Here's how the part is built. I have some questions about the finished solid (model axes, mm). A direction names the side the tool comes from. Give positions to 0.01 mm unless a question says otherwise; leave off trailing zeros. Loops run counter-clockwise (first coordinate to the right, second up) from the corner with the lowest first, then second, coordinate; pieces in that order, holes last. Notation, with made-up numbers: (5, -14) - (47, -14) arc R24 ccw to (47, -3) - close; hole circle Ø3 at (9.5, -26). An arc over 180 degrees is marked (long way). Use a Markdown table: item, result.
Autodesk Inventor part; units mm, degrees
ref_plane "YZ Plane" through (0, 0, 0) normal (1, 0, 0) x (0, 1, 0)
ref_plane "XZ Plane" through (0, 0, 0) normal (0, 1, 0) x (-1, 0, 0)
ref_plane "XY Plane" through (0, 0, 0) normal (0, 0, 1) x (1, 0, 0)
sketch "Sketch1" plane through (0, 0, 0) normal (0, 1, 0) x (-1, 0, 0)
  line L0 (0, 0) -> (11.684, 0)
  line L1 (11.684, 0) -> (11.684, -6.096)
  line L2 (11.684, -6.096) -> (0, -6.096)
  line L3 (0, -6.096) -> (0, -17.78)
  line L4 (0, -17.78) -> (-6.096, -17.78)
  line L5 (-6.096, -17.78) -> (-6.096, -6.096)
  line L6 (-6.096, -6.096) -> (-17.78, -6.096)
  line L7 (-17.78, -6.096) -> (-17.78, 0)
  line L8 (-17.78, 0) -> (-6.096, 0)
  line L9 (-6.096, 0) -> (-6.096, 11.684)
  line L10 (-6.096, 11.684) -> (0, 11.684)
  line L11 (0, 11.684) -> (0, 0)
  arc A0 (11.684, -6.096) -> (11.684, 0) centre (11.684, -3.048) ccw
  arc A1 (-6.096, -17.78) -> (0, -17.78) centre (-3.048, -17.78) ccw
  arc A2 (-17.78, 0) -> (-17.78, -6.096) centre (-17.78, -3.048) ccw
  arc A3 (0, 11.684) -> (-6.096, 11.684) centre (-3.048, 11.684) ccw
  dimension "d0" = 11.684
  dimension "d1" = 6.096
  dimension "d2" = 11.684
  dimension "d3" = 6.096
  dimension "d4" = 11.684
  dimension "d5" = 11.684
extrude "Extrusion1" add sketch "Sketch1" along normal blind 4.2418
properties part number "Part7 x 2"
(1) If I drill on line 1 (X direction, y = 3.75, z = 4); line 2 (Z direction, x = -11.5, y = 3.1); line 3 (Z direction, x = 2, y = 3), over which ranges is the centre line in solid material (lowest first)?
A:
| item | result |
|---|---|
| line 1 | 0 to 6.1 |
| line 2 | -6.1 to 0 |
| line 3 | -20.64 to 14.55 |
(2) Suppose I cut it at A-A on y = 3.35. Write out the boundary of the cut face in (x, z), plus the area to 3 significant figures.
A:
| item | result |
|---|---|
| outline | (-11.68, -6.1) - (0, -6.1) - (0, -17.78) arc R3.05 ccw to (6.1, -17.78) - (6.1, -6.1) - (17.78, -6.1) arc R3.05 ccw to (17.78, 0) - (6.1, 0) - (6.1, 11.68) arc R3.05 ccw to (0, 11.68) - (0, 0) - (-11.68, 0) arc R3.05 ccw to start |
| area | 380 mm2 |
(3) Will these pins go through, and if not, where does the flat tip stop? pin 1 (2 mm diameter, centred on y = 2.5, z = -14.5, fed in from -X); pin 2 (2 mm diameter, centred on y = 1, z = -12.5, fed in from +X); pin 3 (2 mm diameter, centred on x = 10, y = 1.5, fed in from +Z).
A:
| item | result |
|---|---|
| pin 1 | x = 0 |
| pin 2 | x = 6.1 |
| pin 3 | z = 0 |
(4) Suppose I cut it at B-B on z = 8. Write out the boundary of the cut face in (x, y).
A:
| item | result |
|---|---|
| outline | (0, 0) - (6.1, 0) - (6.1, 4.24) - (0, 4.24) - close |
(5) On a 3-axis mill with a long thin cutter (end or side, diameter ignored), from which of +Z, -Z, +X, -X, +Y, -Y can I reach the whole of each face in a straight line? I mean faces 1 (the face through (-6, 2, -6.096)), 2 (the face through (12, 2, -6.096)), 3 (the face through (3.12, 2.09, 14.73)), 4 (the face through (6.096, 2, 6)), 5 (the face through (0, 2, 6)). Say none if no direction works.
A:
| item | result |
|---|---|
| face 1 | -Z, -X, +Y, -Y |
| face 2 | -Z, +X, +Y, -Y |
| face 3 | +Z, +Y, -Y |
| face 4 | +Z, +X, +Y, -Y |
| face 5 | +Z, -X, +Y, -Y |
(6) Suppose I cut it at C-C on x = 1. Write out the boundary of the cut face in (y, z), plus the area to 3 significant figures.
A:
| item | result |
|---|---|
| outline | (0, -20.04) - (4.24, -20.04) - (4.24, 13.94) - (0, 13.94) - close |
| area | 144 mm2 |
